```python
from build123d import *

# Parameters (mm, degrees)
EXTRUDE_1_DEPTH          = 3
SKETCH_3_W               = 19
SKETCH_3_H               = 22
SKETCH_3_H_2             = 19
CUT_EXTRUDE_1_DEPTH      = 3
FILLET_1_R               = 1
FILLET_2_R               = 2
SKETCH_4_R               = 2.025
CUT_EXTRUDE_2_DEPTH      = 3
SKETCH_5_R               = 2.025
CUT_EXTRUDE_3_DEPTH      = 10
EXTRUDE_2_DEPTH          = 3
FILLET_3_R               = 3
SKETCH_8_R               = 1.525
CUT_EXTRUDE_4_DEPTH      = 1
CUT_EXTRUDE_4_DEPTH_BACK = 4


with BuildPart() as part:
    # 草图1 → 凸台-拉伸1 (new body)
    with BuildSketch(Plane.XY):
        Polygon((0, 0), (-70, 0), (-70, 20), (-55, 90), (-15, 90), (0, 20), align=None)
    extrude(amount=EXTRUDE_1_DEPTH)

    # 草图3 → 切除-拉伸1 (cut)
    with BuildSketch(Plane.XY.offset(3)):
        with Locations((-35, 67)):
            Rectangle(SKETCH_3_W, SKETCH_3_H)
        with Locations((-35, 37.5)):
            Rectangle(SKETCH_3_W, SKETCH_3_H_2)
        Polygon((-4.090806018, 20), (-15, 70.909571916), (-15, 20), align=None)
    extrude(amount=-CUT_EXTRUDE_1_DEPTH, mode=Mode.SUBTRACT)

    # 圆角1
    fillet_1_edges = [part.edges().sort_by_distance(p)[0] for p in [
        (-4.090806018, 20, 1.5),
        (-15, 20, 1.5),
        (-15, 70.909571916, 1.5),
    ]]
    fillet(fillet_1_edges, radius=FILLET_1_R)

    # 圆角2
    fillet_2_edges = [part.edges().sort_by_distance(p)[0] for p in [
        (-25.5, 47, 1.5),
        (-25.5, 28, 1.5),
        (-44.5, 28, 1.5),
        (-44.5, 47, 1.5),
        (-25.5, 78, 1.5),
        (-25.5, 56, 1.5),
        (-44.5, 56, 1.5),
        (-44.5, 78, 1.5),
    ]]
    fillet(fillet_2_edges, radius=FILLET_2_R)

    # 草图4 → 切除-拉伸2 (cut)
    with BuildSketch(Plane.XY.offset(3)):
        with Locations((-62.5, 10)):
            Circle(SKETCH_4_R)
        with Locations((-35, 10)):
            Circle(SKETCH_4_R)
        with Locations((-7.5, 10)):
            Circle(SKETCH_4_R)
    extrude(amount=-CUT_EXTRUDE_2_DEPTH, mode=Mode.SUBTRACT)

    # 草图5 → 切除-拉伸3 (cut)
    with BuildSketch(Plane(origin=(0, 0, 0), x_dir=(-1, 0, 0), z_dir=(0, 0, -1))):
        with Locations((35, 82.566965626)):
            Circle(SKETCH_5_R)
        with Locations((35, 51.566965626)):
            Circle(SKETCH_5_R)
        with Locations((35, 24)):
            Circle(SKETCH_5_R)
    extrude(amount=-CUT_EXTRUDE_3_DEPTH, mode=Mode.SUBTRACT)

    # 草图7 → 凸台-拉伸2 (add)
    with BuildSketch(Plane.XY.offset(3)):
        Polygon((-55, 90), (-70, 90), (-70, 20), align=None)
    extrude(amount=-EXTRUDE_2_DEPTH)

    # 圆角3
    fillet_3_edges = [part.edges().sort_by_distance(p)[0] for p in [
        (0, 0, 1.5),
        (-70, 0, 1.5),
        (-15, 90, 1.5),
        (0, 20, 1.5),
        (-70, 90, 1.5),
    ]]
    fillet(fillet_3_edges, radius=FILLET_3_R)

    # 草图8 → 切除-拉伸4 (cut, two sides)
    with BuildSketch(Plane.XY.offset(3)) as cut_extrude_4_sk:
        with Locations((-63.5, 86.5)):
            Circle(SKETCH_8_R)
        with Locations((-63.5, 60.5)):
            Circle(SKETCH_8_R)
        with Locations((-63.5, 51.5)):
            Circle(SKETCH_8_R)
        with Locations((-63.5, 25.5)):
            Circle(SKETCH_8_R)
    extrude(amount=CUT_EXTRUDE_4_DEPTH, mode=Mode.SUBTRACT)
    extrude(cut_extrude_4_sk.sketch, amount=-CUT_EXTRUDE_4_DEPTH_BACK, mode=Mode.SUBTRACT)


solid = part.part
```
The listing builds one solid part. Answer for the finished solid, in the listing's coordinates (mm). A direction names the side the tool comes from. Coordinates: 2 decimals unless noted, no trailing zeros. Loops run counter-clockwise (first coordinate to the right, second up) from the corner with the lowest first, then second, coordinate; pieces in that order, holes last. Notation, with made-up numbers: M -31.75,57.25 L 21.25,57.25 A24 ccw 21.25,93.25 Z; hole C 44.25,-8.75 d5. An arc over 180 degrees is marked long. Answer as CSV lines item,"result". Start each with the question number.
(1) For faces 1 (the flat face through (-70, 46, 2)), 2 (the flat face through (-25.5, 67, 2)), determine the directions among +Z, -Z, +X, -X, +Y, -Y from which every point of the face is accessible in a straight line to the end or side of a thin tool.
(2) The part is cut by section D-D (y = 75). Give the vertices of the cut face in (x, z), and give its area (3 significant figures).
(3) The part is cut by section A-A (y = 10). Give the vertices of the cut face in (x, z) (3 decimals), and give its area (3 significant figures).
(4) The mould has two halves that part along Y. Classify faces 3 (the cylindrical face through (-26.1, 77.43, 1.48)), 4 (the flat face through (0, 11, 1)), 5 (the flat face through (-7.38, 54.44, 1.48)): pulls with the +Y half, pulls with the -Y half, needs draft (parallel to the pull), parting line crosses it, or undercut.
(5) The part is cut by section B-B (x = -28.5). Give the vertices of the cut face in (y, z), and give its area (3 significant figures).
(6) The part is cut by section C-C (x = -63). Give the vertices of the cut face in (y, z), and give its area (3 significant figures).
(7) Find the intervals of material crossed by L1, parallel to Y at x = -41.5, z = 1.8; L2, parallel to Y at x = -63.5, z = 1.1 (3 decimals); L3, parallel to X at y = 44.5, z = 0.3, in increasing order. Write a range as [from, to].
Determined:
1,face 1,"+Z, -Z, -X, +Y, -Y"
1,face 2,"+Z, -Z"
2,outline,"M -70,0 L -44.5,0 L -44.5,3 L -70,3 Z; M -25.5,0 L -11.79,0 L -11.79,3 L -25.5,3 Z"
2,area,"118 mm2"
3,outline,"M -70,0 L -64.525,0 L -64.525,3 L -70,3 Z; M -60.475,0 L -37.025,0 L -37.025,3 L -60.475,3 Z; M -32.975,0 L -9.525,0 L -9.525,3 L -32.975,3 Z; M -5.475,0 L 0,0 L 0,3 L -5.475,3 Z"
3,area,"174 mm2"
4,face 3,"undercut"
4,face 4,"needs draft"
4,face 5,"pulls with the +Y half"
5,outline,"M 0,0 L 28,0 L 28,3 L 0,3 Z; M 47,0 L 56,0 L 56,3 L 47,3 Z; M 78,0 L 90,0 L 90,3 L 78,3 Z"
5,area,"147 mm2"
6,outline,"M 0,0 L 8.04,0 L 8.04,3 L 0,3 Z; M 11.96,0 L 24.06,0 L 24.06,3 L 11.96,3 Z; M 26.94,0 L 50.06,0 L 50.06,3 L 26.94,3 Z; M 52.94,0 L 59.06,0 L 59.06,3 L 52.94,3 Z; M 61.94,0 L 85.06,0 L 85.06,3 L 61.94,3 Z; M 87.94,0 L 90,0 L 90,3 L 87.94,3 Z"
6,area,"224 mm2"
7,L1,"[0, 28], [47, 56], [78, 90]"
7,L2,"[0, 8.239], [11.761, 23.975], [27.025, 49.975], [53.025, 58.975], [62.025, 84.975], [88.025, 90]"
7,L3,"[-70, -44.5], [-25.5, -15], [-9.34, -5.25]"
